Source: CAD feature listing. Evaluate the final solid. Frame: model axes, mm. A direction names the side the tool comes from. Coordinates: 2 decimals unless noted, no trailing zeros. Loops run counter-clockwise (first coordinate to the right, second up) from the corner with the lowest first, then second, coordinate; pieces in that order, holes last.
Item 1: Pin query (flat end, axial travel): pin 1 Ø12 at (x, z) = (22, 23.5) entering from -Y; pin 2 Ø8 at (y, z) = (7, 20) entering from +X; pin 3 Ø2.5 at (x, y) = (-0.3, -29.7) entering from +Z; pin 4 Ø5 at (x, y) = (-22, 9.5) entering from +Z. Return the tip coordinate at first contact, or that it passes through.
Item 2: Section query C-C, the plane x = 24.5. Return the cut outline in (y, z).
Item 3: Pull-direction query (X, two-part tool) for faces 4 (the flat face through (21.3, -36.2, 14.8)), 5 (the cylindrical face through (5.861, 34.526, 17.675)); classes: +X half, -X half, draft (parallel to the pull), parting line (faces both ways), or undercut.
Item 4: Reachability of faces 1 (the cylindrical face through (-64.195, 35.208, 17.675)), 2 (the cylindrical face through (-35.78, -53.69, 19.15)), 3 (the flat face through (-64, -36, 5)) from +Z, -Z, +X, -X, +Y, -Y: full face, straight path, thin tool, end or side. Return the list, or none.
Item 5: Section query A-A, the plane x = -30. State how many separate pieces and enclosed holes the cut face has, then the cut area to 3 significant figures.
Item 6: Line query: probe 1 along Y at (x, z) = (3.5, 20.5); probe 2 along Y at (x, z) = (30, 5.9); probe 3 along Y at (x, z) = (-64.5, 10.25). Output: solid intervals per line, ascending.
Item 7: Section query B-B, the plane y = 14. Return the cut outline in (x, z).
```python
from build123d import *

# Parameters (mm, degrees)
BOSS_EXTRUDE1_DEPTH = 30
SKETCH3_R           = 1.55
CUT_EXTRUDE1_DEPTH  = 22
CUT_EXTRUDE2_START  = -30
SKETCH5_R           = 1.55
CUT_EXTRUDE2_DEPTH  = 30
CUT_EXTRUDE3_START  = -5
SKETCH6_R           = 3.5
CUT_EXTRUDE3_DEPTH  = 5
SKETCH7_R           = 8.2
CUT_EXTRUDE10_DEPTH = 5
SKETCH8_R           = 5
SKETCH8_R_2         = 1.05
CUT_EXTRUDE7_DEPTH  = 8
SKETCH9_R           = 2.2
CUT_EXTRUDE8_DEPTH  = 2.5
SKETCH11_R          = 1.55
CUT_EXTRUDE11_DEPTH = 8
SKETCH12_R          = 3.5
CUT_EXTRUDE12_DEPTH = 3


with BuildPart() as part:
    # Sketch1 → Boss-Extrude1 (new body)
    with BuildSketch(Plane.XY):
        with BuildLine():
            Line((-1.5, 49.363448016), (43.5, 23.382685902))
            ThreePointArc((43.5, 23.382685902), (57, 0), (43.5, -23.382685902))
            Line((43.5, -23.382685902), (-1.5, -49.363448016))
            ThreePointArc((-1.5, -49.363448016), (-87, 0), (-1.5, 49.363448016))
        make_face()
    extrude(amount=BOSS_EXTRUDE1_DEPTH)

    # Sketch3 → Cut-Extrude1 (cut)
    with BuildSketch(Plane.XY.offset(30)):
        with Locations((50.449984706, 0.025940866)):
            Circle(SKETCH3_R)
        with Locations((-80.45, 0)):
            Circle(SKETCH3_R)
        with Locations((-65.673537111, 35.673537111)):
            Circle(SKETCH3_R)
        with Locations((-65.673537111, -35.673537111)):
            Circle(SKETCH3_R)
        with Locations((6.062445841, 36.062445841)):
            Circle(SKETCH3_R)
        with Locations((6.062445841, -36.062445841)):
            Circle(SKETCH3_R)
        with BuildLine():
            Line((-3, -46.765371804), (5.400248357, -41.915486154))
            Line((5.400248357, -41.915486154), (3.031356927, -37.812445841))
            ThreePointArc((3.031356927, -37.812445841), (4.312445841, -33.031356927), (9.093534754, -34.312445841))
            Line((9.093534754, -34.312445841), (11.462426183, -38.415486154))
            Line((11.462426183, -38.415486154), (42, -20.784609691))
            ThreePointArc((42, -20.784609691), (49.859000377, -13.476650327), (53.747229589, -3.474059134))
            Line((53.747229589, -3.474059134), (50.449984706, -3.474059134))
            ThreePointArc((50.449984706, -3.474059134), (46.949984706, 0.025940866), (50.449984706, 3.525940866))
            Line((50.449984706, 3.525940866), (53.739581736, 3.525940866))
            ThreePointArc((53.739581736, 3.525940866), (49.844264614, 13.498339229), (42, 20.784609691))
            Line((42, 20.784609691), (11.462426183, 38.415486154))
            Line((11.462426183, 38.415486154), (9.093534754, 34.312445841))
            ThreePointArc((9.093534754, 34.312445841), (4.312445841, 33.031356927), (3.031356927, 37.812445841))
            Line((3.031356927, 37.812445841), (5.400248357, 41.915486154))
            Line((5.400248357, 41.915486154), (-3, 46.765371804))
            ThreePointArc((-3, 46.765371804), (-35.308766962, 53.738412643), (-65.628603797, 40.578351266))
            Line((-65.628603797, 40.578351266), (-63.198663377, 38.148410845))
            ThreePointArc((-63.198663377, 38.148410845), (-63.198663377, 33.198663377), (-68.148410845, 33.198663377))
            Line((-68.148410845, 33.198663377), (-70.578351266, 35.628603797))
            ThreePointArc((-70.578351266, 35.628603797), (-79.889494756, 20.664905348), (-83.886454699, 3.5))
            Line((-83.886454699, 3.5), (-80.45, 3.5))
            ThreePointArc((-80.45, 3.5), (-76.95, 0), (-80.45, -3.5))
            Line((-80.45, -3.5), (-83.886454699, -3.5))
            ThreePointArc((-83.886454699, -3.5), (-79.889494756, -20.664905348), (-70.578351266, -35.628603797))
            Line((-70.578351266, -35.628603797), (-68.148410845, -33.198663377))
            ThreePointArc((-68.148410845, -33.198663377), (-63.198663377, -33.198663377), (-63.198663377, -38.148410845))
            Line((-63.198663377, -38.148410845), (-65.628603797, -40.578351266))
            ThreePointArc((-65.628603797, -40.578351266), (-35.308766962, -53.738412643), (-3, -46.765371804))
        make_face()
    extrude(amount=-CUT_EXTRUDE1_DEPTH, mode=Mode.SUBTRACT)

    # Sketch5 → Cut-Extrude2 (cut)
    with BuildSketch(Plane(origin=(0, 0, 0), x_dir=(-1, 0, 0), z_dir=(0, 0, -1)).offset(CUT_EXTRUDE2_START)):
        with Locations(Location((80.45, 0, 0), (0, 0, 180))):
            Circle(SKETCH5_R)
        with Locations(Location((-50.449984706, 0.025940866, 0), (0, 0, 180))):
            Circle(SKETCH5_R)
        with Locations(Location((-6.062445841, -36.062445841, 0), (0, 0, 180))):
            Circle(SKETCH5_R)
        with Locations(Location((-6.062445841, 36.062445841, 0), (0, 0, 180))):
            Circle(SKETCH5_R)
        with Locations(Location((65.673537111, 35.673537111, 0), (0, 0, 180))):
            Circle(SKETCH5_R)
        with Locations(Location((65.673537111, -35.673537111, 0), (0, 0, 180))):
            Circle(SKETCH5_R)
    extrude(amount=CUT_EXTRUDE2_DEPTH, mode=Mode.SUBTRACT)

    # Sketch6 → Cut-Extrude3 (cut)
    with BuildSketch(Plane(origin=(0, 0, 0), x_dir=(-1, 0, 0), z_dir=(0, 0, -1)).offset(CUT_EXTRUDE3_START)):
        with Locations((-50.449984706, 0.025940866)):
            Circle(SKETCH6_R)
        with Locations((80.45, 0)):
            Circle(SKETCH6_R)
        with Locations((65.673537111, 35.673537111)):
            Circle(SKETCH6_R)
        with Locations((-6.062445841, 36.062445841)):
            Circle(SKETCH6_R)
        with Locations((65.673537111, -35.673537111)):
            Circle(SKETCH6_R)
        with Locations((-6.062445841, -36.062445841)):
            Circle(SKETCH6_R)
    extrude(amount=CUT_EXTRUDE3_DEPTH, mode=Mode.SUBTRACT)

    # Sketch7 → Cut-Extrude10 (cut)
    with BuildSketch(Plane.XY.offset(8)):
        with Locations((-30, 0)):
            Circle(SKETCH7_R)
        with Locations((30, 0)):
            Circle(SKETCH7_R)
    extrude(amount=-CUT_EXTRUDE10_DEPTH, mode=Mode.SUBTRACT)

    # Sketch8 → Cut-Extrude7 (cut)
    with BuildSketch(Plane.XY.offset(8)):
        with Locations((-30, 0)):
            Circle(SKETCH8_R)
        with Locations((-38.980256121, 8.980256121)):
            Circle(SKETCH8_R_2)
        with Locations((-21.019743879, 8.980256121)):
            Circle(SKETCH8_R_2)
        with Locations((-21.019743879, -8.980256121)):
            Circle(SKETCH8_R_2)
        with Locations((-38.980256121, -8.980256121)):
            Circle(SKETCH8_R_2)
    extrude(amount=-CUT_EXTRUDE7_DEPTH, mode=Mode.SUBTRACT)

    # Sketch9 → Cut-Extrude8 (cut)
    with BuildSketch(Plane.XY.offset(8)):
        with Locations((-38.980256121, 8.980256121)):
            Circle(SKETCH9_R)
        with Locations((-21.019743879, 8.980256121)):
            Circle(SKETCH9_R)
        with Locations((-21.019743879, -8.980256121)):
            Circle(SKETCH9_R)
        with Locations((-38.980256121, -8.980256121)):
            Circle(SKETCH9_R)
    extrude(amount=-CUT_EXTRUDE8_DEPTH, mode=Mode.SUBTRACT)

    # Sketch11 → Cut-Extrude11 (cut)
    with BuildSketch(Plane.XY.offset(8)):
        with Locations((-0.30151519, 29.69848481)):
            Circle(SKETCH11_R)
        with Locations((-30, 42)):
            Circle(SKETCH11_R)
        with Locations((-59.69848481, 29.69848481)):
            Circle(SKETCH11_R)
        with Locations((-72, 0)):
            Circle(SKETCH11_R)
        with Locations((-59.69848481, -29.69848481)):
            Circle(SKETCH11_R)
        with Locations((-30, -42)):
            Circle(SKETCH11_R)
        with Locations((-0.30151519, -29.69848481)):
            Circle(SKETCH11_R)
        with Locations((30, 19)):
            Circle(SKETCH11_R)
        with Locations((30, -19)):
            Circle(SKETCH11_R)
        with Locations((42, 0)):
            Circle(SKETCH11_R)
    extrude(amount=-CUT_EXTRUDE11_DEPTH, mode=Mode.SUBTRACT)

    # Sketch12 → Cut-Extrude12 (cut)
    with BuildSketch(Plane.XY.offset(8)):
        with Locations((-0.30151519, 29.69848481)):
            Circle(SKETCH12_R)
        with Locations((-30, 42)):
            Circle(SKETCH12_R)
        with Locations((-59.69848481, 29.69848481)):
            Circle(SKETCH12_R)
        with Locations((-72, 0)):
            Circle(SKETCH12_R)
        with Locations((-59.69848481, -29.69848481)):
            Circle(SKETCH12_R)
        with Locations((-30, -42)):
            Circle(SKETCH12_R)
        with Locations((-0.30151519, -29.69848481)):
            Circle(SKETCH12_R)
        with Locations((30, 19)):
            Circle(SKETCH12_R)
        with Locations((42, 0)):
            Circle(SKETCH12_R)
        with Locations((30, -19)):
            Circle(SKETCH12_R)
    extrude(amount=-CUT_EXTRUDE12_DEPTH, mode=Mode.SUBTRACT)


solid = part.part
```
Verdict:
1. pin 1: stops at y = -39.26
1. pin 2: stops at x = 56.83
1. pin 3: passes through
1. pin 4: stops at z = 8
2. outline: (-34.35, 0) - (34.35, 0) - (34.35, 30) - (30.89, 30) - (30.89, 8) - (6.08, 8) - (6.08, 3) - (-6.08, 3) - (-6.08, 8) - (-30.89, 8) - (-30.89, 30) - (-34.35, 30) - close
3. face 4: +X half
3. face 5: undercut
4. face 1: +Z, -Z
4. face 2: +Z
4. face 3: -Z
5. separate pieces: 4
5. enclosed holes: 0
5. area: 859 mm2
6. probe 1: y = -46.48 to -43.01, -38.62 to -33.68, 33.68 to 38.62, 43.01 to 46.48
6. probe 2: y = -31.18 to -22.5, -15.5 to -8.2, 8.2 to 15.5, 22.5 to 31.18
6. probe 3: y = -45.37 to -41.54, -39.45 to -36.69, -34.66 to -32.38, 32.38 to 34.66, 36.69 to 39.45, 41.54 to 45.37
7. outline: (-85.25, 0) - (53.09, 0) - (53.09, 30) - (49.49, 30) - (49.49, 8) - (-82.15, 8) - (-82.15, 30) - (-85.25, 30) - close
